Build history of the part. All positions in model axes, mm. Face numbers are marked on the shaded views. A direction names the side the tool comes from. Give positions to 0.01 mm unless a question says otherwise; leave off trailing zeros. Write each loop counter-clockwise with the first axis right and the second up, starting at its lowest first coordinate (ties: lowest second). Pieces come first, ordered by that corner, then holes. Notation, with made-up numbers: (67, -35) -> (99, -35) arc R24 ccw to (99, -22) -> close; hole circle Ø6 at (28.5, 69). An arc over 180 degrees is marked (long way). Put each result on its own line as item: value. Start each with the question number.
Item 1: Slice it at B-B, the plane y = 0. List the corners of the cut face in (x, z), plus the area to 3 significant figures.
Item 2: Drill centre lines: line 1 along Y through (x, z) = (0, 70.5); line 2 along Z through (x, y) = (6.5, 5.25); line 3 along Z through (x, y) = (-2.25, -4.5). Where is each one in solid material? Low to high.
Item 3: Slice it at A-A, the plane x = 0. List the corners of the cut face in (y, z).
Item 4: Slice it at D-D, the plane x = -7. List the corners of the cut face in (y, z).
Item 5: Slice it at C-C, the plane z = 93.5. List the corners of the cut face in (x, y), plus the area to 3 significant figures.
Item 6: Tool access for the marked faces 1 and 2: list every direction of +Z, -Z, +X, -X, +Y, -Y with a clear straight run to the whole face (end or side of a thin tool).
Item 7: Flat gauge pins, fed straight in: pin 1 Ø3 at (x, z) = (-4.5, 74) entering from +Y; pin 2 Ø6 at (y, z) = (-2, 31) entering from +X; pin 3 Ø6 at (y, z) = (4, 43) entering from -X. Where does each tip first touch, or does it go through?
```python
from build123d import *

# Parameters (mm, degrees)
F0_R     = 8.5
F1_DEPTH = 4
F2_R     = 5
F3_DEPTH = 100
F4_W     = 4
F4_H     = 5
F6_W     = 4
F6_H     = 36.891641
F7_DEPTH = 1
F8_R     = 1.5
F9_DEPTH = 122


with BuildPart() as f1:
    # F0 (on Top) → F1 (new body)
    with BuildSketch(Plane.XY):
        Circle(F0_R)
    extrude(amount=F1_DEPTH)

    # F2 (on Top) → F3 (join)
    with BuildSketch(Plane.XY):
        Circle(F2_R)
    extrude(amount=F3_DEPTH)

    # F4 (on Right) → F5 (revolve)
    with BuildSketch(Plane.YZ):
        with Locations((2, 102.5)):
            Rectangle(F4_W, F4_H)
    revolve(axis=Axis((0, 0, 102.5), (0, 0, -1)))

    # F6 (on face) → F7 (cut)
    with BuildSketch(Plane(origin=(0, 0, 0), x_dir=(1, 0, 0), z_dir=(0, 0, -1))):
        with Locations((6, -0.745802)):
            Rectangle(F6_W, F6_H)
    extrude(amount=-F7_DEPTH, mode=Mode.SUBTRACT)

    # F8 (on face) → F9 (cut)
    with BuildSketch(Plane.XY.offset(105)):
        Circle(F8_R)
    extrude(amount=-F9_DEPTH, mode=Mode.SUBTRACT)


solid = f1.part
```
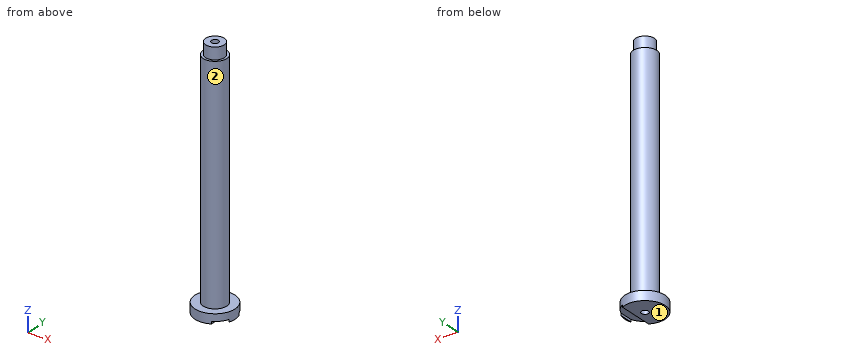
Values follow:
1. outline: (-8.5, 0) -> (-1.5, 0) -> (-1.5, 105) -> (-4, 105) -> (-4, 100) -> (-5, 100) -> (-5, 4) -> (-8.5, 4) -> close; (1.5, 0) -> (4, 0) -> (4, 1) -> (8, 1) -> (8, 0) -> (8.5, 0) -> (8.5, 4) -> (5, 4) -> (5, 100) -> (4, 100) -> (4, 105) -> (1.5, 105) -> close
1. area: 749 mm2
2. line 1: -5 to -1.5, 1.5 to 5
2. line 2: 1 to 4
2. line 3: 0 to 4
3. outline: (-8.5, 0) -> (-1.5, 0) -> (-1.5, 105) -> (-4, 105) -> (-4, 100) -> (-5, 100) -> (-5, 4) -> (-8.5, 4) -> close; (1.5, 0) -> (8.5, 0) -> (8.5, 4) -> (5, 4) -> (5, 100) -> (4, 100) -> (4, 105) -> (1.5, 105) -> close
4. outline: (-4.82, 0) -> (4.82, 0) -> (4.82, 4) -> (-4.82, 4) -> close
5. outline: circle Ø10 at (0, 0); hole circle Ø3 at (0, 0)
5. area: 71.5 mm2
6. face 1: -Z, +X, -X, +Y, -Y
6. face 2: +Z
7. pin 1: y = 4
7. pin 2: x = 5
7. pin 3: x = -4.9
